from build123d import *

# Parameters (mm, degrees)
SKETCH1_W           = 14.011388394
SKETCH1_H           = 5.937625438
SKETCH1_R           = 1.15
SKETCH1_R_2         = 1.35
SKETCH1_R_3         = 1.85
BOSS_EXTRUDE1_DEPTH = 2


with BuildPart() as part:
    # Sketch1 → Boss-Extrude1 (new body)
    with BuildSketch(Plane(origin=(0, 0, 0), x_dir=(1, 0, 0), z_dir=(0, 1, 0))):
        Rectangle(SKETCH1_W, SKETCH1_H)
        with Locations((-3.653842684, 0)):
            Circle(SKETCH1_R, mode=Mode.SUBTRACT)
        Circle(SKETCH1_R_2, mode=Mode.SUBTRACT)
        with Locations((4.147880665, 0)):
            Circle(SKETCH1_R_3, mode=Mode.SUBTRACT)
    extrude(amount=BOSS_EXTRUDE1_DEPTH)


solid = part.part
Verification items for the finished model (mm, model axes). Round coordinates to 2 decimals unless told otherwise and drop trailing zeros. Order: outer loops, then holes, each group sorted by start corner. A loop starts at its lowest first (then second) coordinate and runs counter-clockwise, first axis right, second up.
1. Section check D-D on z = 1.55. Record the cut outline in (x, y).
Final values:
outline: (-7.01, 0) - (3.14, 0) - (3.14, 2) - (-7.01, 2) - close; (5.16, 0) - (7.01, 0) - (7.01, 2) - (5.16, 2) - close
2. Section check B-B on x = 0. Record the cut outline in (y, z), then the cut area to 3 significant figures.
Final values:
outline: (0, -2.97) - (2, -2.97) - (2, -1.35) - (0, -1.35) - close; (0, 1.35) - (2, 1.35) - (2, 2.97) - (0, 2.97) - close
area: 6.48 mm2
3. Release check for a two-part mould opening along X. For faces 1 (the flat face through (-7.006, 1, 0)), 2 (the flat face through (0, 1, -2.969)), 3 (the cylindrical face through (-2.59, 0.99, 0.44)) record: +X half, -X half, draft (parallel to the pull), parting line (faces both ways), or undercut.
Final values:
face 1: -X half
face 2: draft
face 3: undercut
4. Section check C-C on y = 0.7. Record the cut outline in (x, z), then the cut area to 3 significant figures.
Final values:
outline: (-7.01, -2.97) - (7.01, -2.97) - (7.01, 2.97) - (-7.01, 2.97) - close; hole circle Ø2.3 at (-3.65, 0); hole circle Ø2.7 at (0, 0); hole circle Ø3.7 at (4.15, 0)
area: 62.6 mm2
5. Thickness scan on L1, parallel to X at y = 1, z = 0; L2, parallel to Z at x = 0, y = 0.5; L3, parallel to X at y = 1.75, z = 0.45. Record the ranges inside material, lowest first.
Final values:
L1: x = -7.01 to -4.8, -2.5 to -1.35, 1.35 to 2.3, 6 to 7.01
L2: z = -2.97 to -1.35, 1.35 to 2.97
L3: x = -7.01 to -4.71, -2.6 to -1.27, 1.27 to 2.35, 5.94 to 7.01
6. Go/stop test with flat-tipped pins: P1, Ø3.5, axis at x = 0, z = 0, coming from the -Y side; P2, Ø2, axis at x = 4.15, z = 0, coming from the -Y side. Record where each tip stops, or that it passes through.
Final values:
P1: stops at y = 0
P2: passes through
7. Section check A-A on z = 0. Record the cut outline in (x, y), then the cut area to 3 significant figures.
Final values:
outline: (-7.01, 0) - (-4.8, 0) - (-4.8, 2) - (-7.01, 2) - close; (-2.5, 0) - (-1.35, 0) - (-1.35, 2) - (-2.5, 2) - close; (1.35, 0) - (2.3, 0) - (2.3, 2) - (1.35, 2) - close; (6, 0) - (7.01, 0) - (7.01, 2) - (6, 2) - close
area: 10.6 mm2
